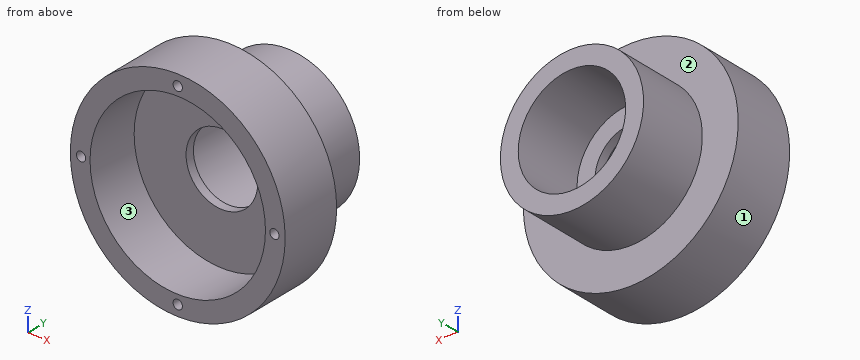
from build123d import *

# Parameters (mm, degrees)
SKETCH1_R           = 38.1
SKETCH1_R_2         = 31.115
BOSS_EXTRUDE1_DEPTH = 19.05
SKETCH2_R           = 1.64973
CUT_EXTRUDE1_DEPTH  = 12.7
SKETCH3_R           = 38.1
SKETCH3_R_2         = 12.7
BOSS_EXTRUDE2_DEPTH = 3.175
SKETCH4_R           = 25.4
SKETCH4_R_2         = 19.05
BOSS_EXTRUDE3_DEPTH = 25.4


with BuildPart() as part:
    # Sketch1 → Boss-Extrude1 (new body)
    with BuildSketch(Plane(origin=(0, 0, 0), x_dir=(1, 0, 0), z_dir=(0, 1, 0))):
        Circle(SKETCH1_R)
        Circle(SKETCH1_R_2, mode=Mode.SUBTRACT)
    extrude(amount=BOSS_EXTRUDE1_DEPTH)

    # Sketch2 → Cut-Extrude1 (cut)
    with BuildSketch(Plane.XZ):
        with Locations((0, 34.29)):
            Circle(SKETCH2_R)
        with Locations((34.29, 0)):
            Circle(SKETCH2_R)
        with Locations((0, -34.29)):
            Circle(SKETCH2_R)
        with Locations((-34.29, 0)):
            Circle(SKETCH2_R)
    extrude(amount=-CUT_EXTRUDE1_DEPTH, mode=Mode.SUBTRACT)

    # Sketch3 → Boss-Extrude2 (add)
    with BuildSketch(Plane(origin=(0, 19.05, 0), x_dir=(1, 0, 0), z_dir=(0, 1, 0))):
        Circle(SKETCH3_R)
        Circle(SKETCH3_R_2, mode=Mode.SUBTRACT)
    extrude(amount=BOSS_EXTRUDE2_DEPTH)

    # Sketch4 → Boss-Extrude3 (add)
    with BuildSketch(Plane(origin=(0, 22.225, 0), x_dir=(1, 0, 0), z_dir=(0, 1, 0))):
        Circle(SKETCH4_R)
        Circle(SKETCH4_R_2, mode=Mode.SUBTRACT)
    extrude(amount=BOSS_EXTRUDE3_DEPTH)


solid = part.part
Model file for the job. Use its own axes, mm. Face numbers are marked on the shaded views. A direction names the side the tool comes from. Coordinates: 2 decimals unless noted, no trailing zeros. Write each loop counter-clockwise with the first axis right and the second up, starting at its lowest first coordinate (ties: lowest second). Pieces come first, ordered by that corner, then holes. Notation, with made-up numbers: (16.5, 8.5) -> (70.5, 8.5) arc R24 ccw to (70.5, 24.5) -> close; hole circle Ø1 at (60.25, 7). An arc over 180 degrees is marked (long way). One line per item, written item: value. Start each with the question number.
1) Slice it at A-A on z = 0. Write the cut outline in (x, y) (3 decimals), then the cut area to 3 significant figures.
2) Probe probe 1 along Z at (x, y) = (0, 3) (3 decimals); probe 2 along Y at (x, z) = (-12, -27.5) (3 decimals); probe 3 along Z at (x, y) = (0, 13.5) (3 decimals). List the from-to ranges inside material, lowest first.
3) Flat gauge pins, fed straight in: pin 1 Ø2 at (x, z) = (2, 15) entering from +Y (3 decimals); pin 2 Ø3 at (y, z) = (12.5, 8.5) entering from +X; pin 3 Ø5 at (x, z) = (9.5, -22.5) entering from -Y. Where does each tip first touch, or does it go through?
4) Slice it at D-D on z = 16.5. Write the cut outline in (x, y) (3 decimals).
5) Which spindle directions (+Z, -Z, +X, -X, +Y, -Y) get a long thin tool onto all of the face, cutting with end or side? Do the marked faces 1, 2 and 3. Say none if no direction does.
6) Slice it at C-C on y = 24. Write the cut outline in (x, z).
7) Slice it at B-B on x = -6. Write the cut outline in (y, z) (3 decimals), then the cut area to 3 significant figures.
Answers follow:
1. outline: (-38.1, 0) -> (-35.94, 0) -> (-35.94, 12.7) -> (-32.64, 12.7) -> (-32.64, 0) -> (-31.115, 0) -> (-31.115, 19.05) -> (-12.7, 19.05) -> (-12.7, 22.225) -> (-19.05, 22.225) -> (-19.05, 47.625) -> (-25.4, 47.625) -> (-25.4, 22.225) -> (-38.1, 22.225) -> close; (12.7, 19.05) -> (31.115, 19.05) -> (31.115, 0) -> (32.64, 0) -> (32.64, 12.7) -> (35.94, 12.7) -> (35.94, 0) -> (38.1, 0) -> (38.1, 22.225) -> (25.4, 22.225) -> (25.4, 47.625) -> (19.05, 47.625) -> (19.05, 22.225) -> (12.7, 22.225) -> close
1. area: 666 mm2
2. probe 1: -38.1 to -35.94, -32.64 to -31.115, 31.115 to 32.64, 35.94 to 38.1
2. probe 2: 19.05 to 22.225
2. probe 3: -38.1 to -31.115, 31.115 to 38.1
3. pin 1: y = 22.225
3. pin 2: x = 37.45
3. pin 3: y = 19.05
4. outline: (-34.342, 0) -> (-26.38, 0) -> (-26.38, 19.05) -> (26.38, 19.05) -> (26.38, 0) -> (34.342, 0) -> (34.342, 22.225) -> (19.311, 22.225) -> (19.311, 47.625) -> (9.521, 47.625) -> (9.521, 22.225) -> (-9.521, 22.225) -> (-9.521, 47.625) -> (-19.311, 47.625) -> (-19.311, 22.225) -> (-34.342, 22.225) -> close
5. face 1: +Y, -Y
5. face 2: +Y
5. face 3: -Y
6. outline: circle Ø50.8 at (0, 0); hole circle Ø38.1 at (0, 0)
7. outline: (0, -37.625) -> (22.225, -37.625) -> (22.225, -24.681) -> (47.625, -24.681) -> (47.625, -18.08) -> (22.225, -18.08) -> (22.225, -11.193) -> (19.05, -11.193) -> (19.05, -30.531) -> (0, -30.531) -> close; (0, 30.531) -> (19.05, 30.531) -> (19.05, 11.193) -> (22.225, 11.193) -> (22.225, 18.08) -> (47.625, 18.08) -> (47.625, 24.681) -> (22.225, 24.681) -> (22.225, 37.625) -> (0, 37.625) -> close
7. area: 773 mm2
